```python
from build123d import *

# Parameters (mm, degrees)
ESQUISSE1_R      = 7
EXTRUSION1_DEPTH = 7


with BuildPart() as part:
    # Esquisse1 → Extrusion1 (new body)
    with BuildSketch(Plane(origin=(0, 0, 0), x_dir=(-1, 0, 0), z_dir=(0, 0, -1))):
        with BuildLine():
            Line((0, 12), (-42, 12))
            ThreePointArc((-42, 12), (-54, 0), (-42, -12))
            Line((-42, -12), (0, -12))
            ThreePointArc((0, -12), (12, 0), (0, 12))
        make_face()
        with Locations(Location((-42, 0, 0), (0, 0, 180))):
            Circle(ESQUISSE1_R, mode=Mode.SUBTRACT)
        with Locations(Location((0, 0, 0), (0, 0, 180))):
            Circle(ESQUISSE1_R, mode=Mode.SUBTRACT)
    extrude(amount=-EXTRUSION1_DEPTH)


solid = part.part
```
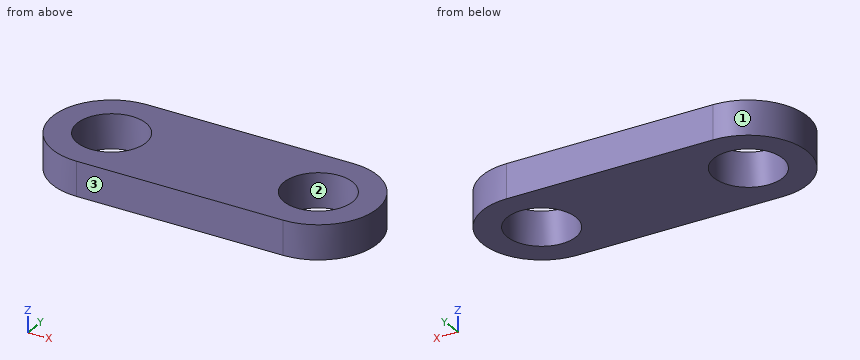
The listing builds one solid part. Answer for the finished solid, in the listing's coordinates (mm). Face numbers are marked on the shaded views. Give positions to 0.01 mm unless a question says otherwise; leave off trailing zeros. Loops run counter-clockwise (first coordinate to the right, second up) from the corner with the lowest first, then second, coordinate; pieces in that order, holes last. Notation, with made-up numbers: M 72,64.25 L 102,64.25 A13 cw 102,78.25 Z; hole C 19,83 d9. An arc over 180 degrees is marked long. One line per item, written item: value.
1. Section B-B on x = 3 is taken. Determine the outline of the cut face in (y, z).
Found:
outline: M -12,0 L -6.32,0 L -6.32,7 L -12,7 Z; M 6.32,0 L 12,0 L 12,7 L 6.32,7 Z
2. This flat-tipped pin is pushed along its axis until it touches: P1, Ø11, axis at x = 0, y = 0, coming from the +Z side. Where does it stop, or does it pass through?
Found:
P1: through
3. Find the intervals of material crossed by probe 1 along Y at (x, z) = (42, 1.5); probe 2 along X at (y, z) = (5, 2.25); probe 3 along X at (y, z) = (1.25, 6.75), in increasing order.
Found:
probe 1: -12 to -7, 7 to 12
probe 2: -10.91 to -4.9, 4.9 to 37.1, 46.9 to 52.91
probe 3: -11.93 to -6.89, 6.89 to 35.11, 48.89 to 53.93
4. For a pull along X with two mould halves and no side action, classify the marked faces 1, 2 and 3 as pulls with the +X half, pulls with the -X half, needs draft (parallel to the pull), parting line crosses it, or undercut.
Found:
face 1: pulls with the -X half
face 2: undercut
face 3: needs draft
5. Section C-C on z = 3.75 is taken. Determine the outline of the cut face in (x, y), plus the area to 3 significant figures.
Found:
outline: M 0,-12 L 42,-12 A12 ccw 42,12 L 0,12 A12 ccw Z; hole C 0,0 d14; hole C 42,0 d14
area: 1,150 mm^2
6. Section A-A on y = 0 is taken. Determine the outline of the cut face in (x, z).
Found:
outline: M -12,0 L -7,0 L -7,7 L -12,7 Z; M 7,0 L 35,0 L 35,7 L 7,7 Z; M 49,0 L 54,0 L 54,7 L 49,7 Z
7. Section D-D on x = 48 is taken. Determine the outline of the cut face in (y, z), plus the area to 3 significant figures.
Found:
outline: M -10.39,0 L -3.61,0 L -3.61,7 L -10.39,7 Z; M 3.61,0 L 10.39,0 L 10.39,7 L 3.61,7 Z
area: 95.0 mm^2
